Geometry check sheet. Reference: the model listing, model coordinates, mm. Give positions to 0.01 mm unless a question says otherwise; leave off trailing zeros. Loops run counter-clockwise (first coordinate to the right, second up) from the corner with the lowest first, then second, coordinate; pieces in that order, holes last. Notation, with made-up numbers: (51.25, -33) -> (80.25, -33) arc R18 cw to (80.25, -4) -> close; hole circle Ø4 at (-3.75, -16.75). An arc over 180 degrees is marked (long way). One line per question, with ' | ' between items.
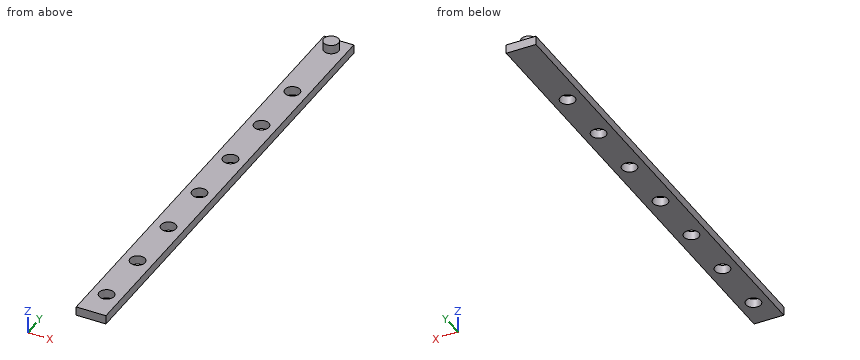
from build123d import *

# Parameters (mm, degrees)
SKETCH_1_W      = 10
SKETCH_1_H      = 160
SKETCH_1_R      = 2.5
EXTRUDE_1_DEPTH = 3
SKETCH_2_R      = 2.5
EXTRUDE_2_DEPTH = 3


with BuildPart() as part:
    # 草圖1 → 填料-伸長1 (new body)
    with BuildSketch(Plane.XY):
        Rectangle(SKETCH_1_W, SKETCH_1_H)
        with Locations((0, -70)):
            Circle(SKETCH_1_R, mode=Mode.SUBTRACT)
        with Locations((0, -50)):
            Circle(SKETCH_1_R, mode=Mode.SUBTRACT)
        with Locations((0, -30)):
            Circle(SKETCH_1_R, mode=Mode.SUBTRACT)
        with Locations((0, -10)):
            Circle(SKETCH_1_R, mode=Mode.SUBTRACT)
        with Locations((0, 10)):
            Circle(SKETCH_1_R, mode=Mode.SUBTRACT)
        with Locations((0, 30)):
            Circle(SKETCH_1_R, mode=Mode.SUBTRACT)
        with Locations((0, 50)):
            Circle(SKETCH_1_R, mode=Mode.SUBTRACT)
    extrude(amount=EXTRUDE_1_DEPTH)

    # 草圖2 → 填料-伸長2 (add)
    with BuildSketch(Plane.XY.offset(3)):
        with Locations(Location((0, 75, 0), (0, 0, 180))):
            Circle(SKETCH_2_R)
    extrude(amount=EXTRUDE_2_DEPTH)


solid = part.part
Item 1: Sectioned sample at C-C (x = -0.5). Give the number of separate pieces and of enclosed holes in the cut face, plus the area to 3 significant figures.
Result:
separate pieces: 8 | enclosed holes: 0 | area: 392 mm2
Item 2: Sectioned sample at B-B (z = 1.85). Record the cut outline in (x, y), plus the area to 3 significant figures.
Result:
outline: (-5, -80) -> (5, -80) -> (5, 80) -> (-5, 80) -> close; hole circle Ø5 at (0, -70); hole circle Ø5 at (0, -50); hole circle Ø5 at (0, -30); hole circle Ø5 at (0, -10); hole circle Ø5 at (0, 10); hole circle Ø5 at (0, 30); hole circle Ø5 at (0, 50) | area: 1,460 mm2
Item 3: Sectioned sample at A-A (y = 10). Record the cut outline in (x, z).
Result:
outline: (-5, 0) -> (-2.5, 0) -> (-2.5, 3) -> (-5, 3) -> close; (2.5, 0) -> (5, 0) -> (5, 3) -> (2.5, 3) -> close
Item 4: Depth check by flat-ended pin: pin 1 Ø1 at (x, y) = (-2, -27.5) entering from +Z. Enter the tip coordinate at first touch or a pass-through.
Result:
pin 1: z = 3
Item 5: Sectioned sample at D-D (y = -36). Record the cut outline in (x, z).
Result:
outline: (-5, 0) -> (5, 0) -> (5, 3) -> (-5, 3) -> close
Item 6: Scan lines: probe 1 along Z at (x, y) = (3, -55); probe 2 along X at (y, z) = (28, 2.75); probe 3 along X at (y, z) = (51.5, 1.05). Record each from-to range of solid material in increasing order.
Result:
probe 1: 0 to 3 | probe 2: -5 to -1.5, 1.5 to 5 | probe 3: -5 to -2, 2 to 5
